Geometry check sheet. Reference: the model listing, model coordinates, mm. Face numbers are marked on the shaded views. A direction names the side the tool comes from. Round coordinates to 2 decimals unless told otherwise and drop trailing zeros. Order: outer loops, then holes, each group sorted by start corner. A loop starts at its lowest first (then second) coordinate and runs counter-clockwise, first axis right, second up.
Autodesk Inventor part; units mm, degrees
ref_plane "YZ Plane" through (0, 0, 0) normal (1, 0, 0) x (0, 1, 0)
ref_plane "XZ Plane" through (0, 0, 0) normal (0, 1, 0) x (-1, 0, 0)
ref_plane "XY Plane" through (0, 0, 0) normal (0, 0, 1) x (1, 0, 0)
sketch "Sketch18" plane through (0, 0, 0) normal (0, 0, 1) x (1, 0, 0)
  circle A0 centre (0, 0) radius 3.302
  circle A1 centre (0, 0) radius 9.525
  line L0 (-9.525, -22.225) -> (53.975, -22.225)
  line L1 (53.975, -22.225) -> (53.975, 9.525)
  line L2 (53.975, 9.525) -> (-9.525, 9.525)
  line L3 (-9.525, 9.525) -> (-9.525, -22.225)
  dimension "d100" = 6.604
  dimension "d101" = 19.05
  dimension "d102" = 63.5
  dimension "d103" = 31.75
extrude "Extrusion17" add sketch "Sketch18" along normal blind 19.05
sketch "Sketch19" plane through (-9.525, -22.225, 0) normal (-1, 0, 0) x (0, 0, 1)
  circle A0 centre (9.525, 9.525) radius 9.525 construction
  circle A1 centre (9.525, 9.525) radius 3.556
  line L0 (0, 31.75) -> (0, 0)
  line L1 (0, 0) -> (19.05, 0)
  point P0 (0, 22.225)
  dimension "d106" = 19.05
  dimension "d107" = 7.112
extrude "Extrusion18" cut sketch "Sketch19" against normal through all
sketch "Sketch20" plane through (0, 0, 19.05) normal (0, 0, 1) x (1, 0, 0)
  line L0 (12.7, -41.275) -> (38.1, -41.275)
  line L1 (38.1, -41.275) -> (38.1, -3.175)
  line L2 (38.1, -3.175) -> (12.7, -3.175)
  line L3 (12.7, -3.175) -> (12.7, -41.275)
  line L4 (-9.525, -22.225) -> (53.975, -22.225)
  line L5 (12.7, -41.275) -> (38.1, -3.175) construction
  line L6 (38.1, -41.275) -> (12.7, -3.175) construction
  circle A0 centre (0, 0) radius 3.302
  point P0 (25.4, -22.225)
  point P1 (12.7, -22.225)
  point P2 (38.1, -22.225)
  dimension "d110" = 25.4
  dimension "d111" = 38.1
  dimension "d112" = 12.7
extrude "Extrusion19" cut sketch "Sketch20" against normal through all contours L3 L2 L1 L4
sketch "Sketch21" plane through (-9.525, -22.225, 0) normal (-1, 0, 0) x (0, 0, 1)
  circle A0 centre (9.525, 9.525) radius 3.556
  circle A1 centre (9.525, 9.525) radius 6.35
  line L0 (3.175, -9.525) -> (15.875, -9.525)
  line L1 (15.875, -9.525) -> (15.875, 9.525)
  line L2 (15.875, 9.525) -> (3.175, 9.525) construction
  line L3 (3.175, 9.525) -> (3.175, -9.525)
  line L4 (19.05, 0) -> (0, 0)
  line L5 (3.175, -9.525) -> (15.875, 9.525) construction
  line L6 (15.875, -9.525) -> (3.175, 9.525) construction
  point P0 (0, 22.225)
  point P1 (9.525, 0)
  point P2 (3.175, 0)
  point P3 (15.875, 0)
  point P4 (3.175, 9.525)
  dimension "d115" = 12.7
extrude "Extrusion20" cut sketch "Sketch21" against normal blind 19.05 contours A1
sketch "Sketch22" plane through (0, 0, 19.05) normal (0, 0, 1) x (1, 0, 0)
  circle A0 centre (0, 0) radius 9.525
  line L0 (-9.525, 9.525) -> (-9.525, -22.225)
  line L1 (9.525, -22.225) -> (-9.525, -22.225)
  line L2 (9.525, -22.225) -> (-6.569, -6.8974)
  line L3 (12.7, -22.225) -> (12.7, -3.175)
  line L4 (53.975, 9.525) -> (-9.525, 9.525)
  point P0 (-9.525, 0)
  point P1 (0, 9.525)
  dimension "d118" = 3.175
extrude "Extrusion21" cut sketch "Sketch22" against normal through all contours L2 L1 L0 A0 | L0 L4 A0
fillet "Fillet12" radius 1.5875 1 edges at (9.525, -12.7, 3.175)
fillet "Fillet13" radius 9.525 4 edges at (11.1125, -22.225, 19.05) (11.1125, -22.225, 0) (46.0375, -22.225, 19.05) (46.0375, -22.225, 0)
sketch "Sketch25" plane through (53.975, 9.525, 19.05) normal (1, 0, 0) x (0, 0, -1)
  line L0 (0, -22.225) -> (0, -12.7)
  line L1 (0, -12.7) -> (12.7, 0)
  line L2 (19.05, 0) -> (0, 0)
  line L3 (0, -22.225) -> (0, 0)
  point P0 (19.05, -9.525)
  dimension "d131" = 6.35
extrude "Extrusion24" cut sketch "Sketch25" against normal through all
sketch "Sketch26" plane through (0, 0, 19.05) normal (0, 0, 1) x (1, 0, 0)
  circle A0 centre (0, 0) radius 6.35
  dimension "d134" = 12.7
extrude "Extrusion25" cut sketch "Sketch26" against normal blind 15.875
fillet "Fillet16" radius 3.175 1 edges at (25.4, -3.175, 19.05)
fillet "Fillet17" radius 6.35 3 edges at (9.0996, -3.175, 19.05) (-7.2398, -3.175, 19.05) (46.0375, -3.175, 19.05)
fillet "Fillet18" radius 1.5875 1 edges at (-6.35, 0, 3.175)
properties part number "Mod Mount" material "UHMW, White"
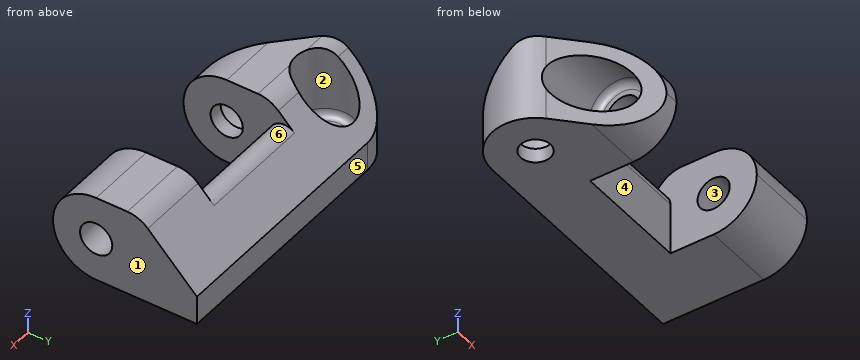
(1) Sectioned sample at B-B, the plane y = -14.5. Give the number of separate pieces and of enclosed holes in the cut face, and give its area (3 significant figures).
Returned:
separate pieces: 4
enclosed holes: 0
area: 294 mm2
(2) Sectioned sample at A-A, the plane x = 15. Record the cut outline in (y, z) (3 decimals).
Returned:
outline: (-3.175, 0) - (9.525, 0) - (9.525, 6.35) - (2.245, 13.63) arc R3.175 ccw to (-3.175, 11.385) - close
(3) Depth check by flat-ended pin: P1, Ø5, axis at y = -11.5, z = 9.5, coming from the -X side (3 decimals); P2, Ø1.5, axis at x = 2, z = 7.5, coming from the -Y side; P3, Ø8, axis at y = -19, z = 15.5, coming from the -X side. Enter the tip coordinate at first touch or a pass-through.
Returned:
P1: stops at x = 9.525
P2: stops at y = -6.99
P3: stops at x = 1.94
(4) Material ranges on line 1 (X direction, y = -4.5, z = 9.25) (3 decimals); line 2 (X direction, y = -3, z = 13) (3 decimals); line 3 (X direction, y = -9, z = 6.25) (3 decimals), recorded low to high.
Returned:
line 1: x = -8.395 to -4.48, 4.48 to 12.7, 38.1 to 53.975
line 2: x = -9.04 to -5.597, 5.597 to 12.7, 38.1 to 53.975
line 3: x = 9.515 to 12.7, 38.1 to 53.975
(5) Set-up check for the marked faces 4, 5 and 6: record each of +Z, -Z, +X, -X, +Y, -Y from which the full face is reachable in a straight line by a thin tool's end or side.
Returned:
face 4: +Z, -Z, -Y
face 5: +Z, -Z, +X, -X, +Y
face 6: +Z
(6) Draft check along X on the marked faces 1, 2 and 3. Enter one of: released by +X, released by -X, zero draft, split by the parting line, or undercut.
Returned:
face 1: released by +X
face 2: undercut
face 3: zero draft
